Answer from the drawing. Dimensions are ordinates in mm from the lowest x, y and z of the part. Round coordinates to 2 decimals unless told otherwise and drop trailing zeros. Loops run counter-clockwise (first coordinate to the right, second up) from the corner with the lowest first, then second, coordinate; pieces in that order, holes last.
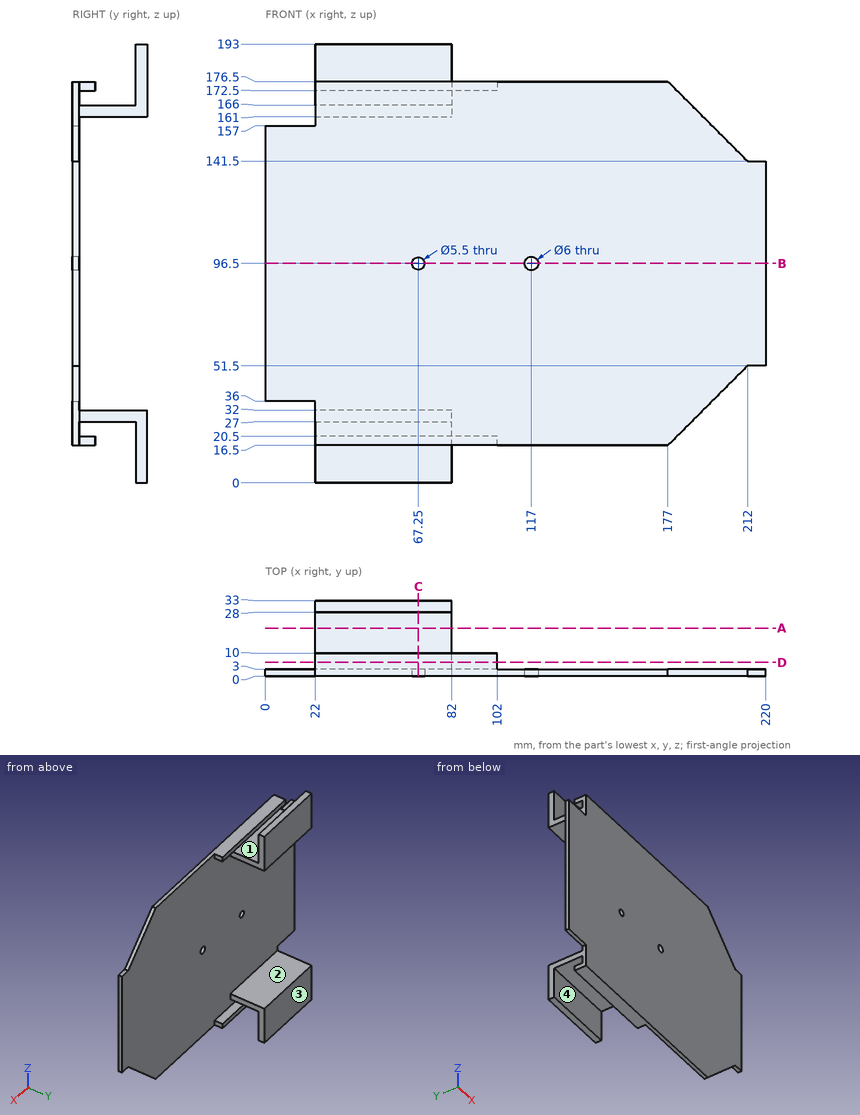
Item 1: Straight lines are drawn through the part: line 1 (Z direction, x = 40, y = 6); line 2 (X direction, y = 2, z = 96); line 3 (Z direction, x = 67.25, y = 1.4). For each, find the intervals that lie inside material, in ascending order.
Item 2: Each of these flat-tipped pins is pushed along its axis until it touches: P1, Ø1.5, axis at x = 217.5, y = 1, coming from the -Z side; P2, Ø1.5, axis at x = 215, y = 1, coming from the +Z side; P3, Ø5, axis at x = 130, y = 4, coming from the +Z side; P4, Ø5, axis at x = 117, z = 96.5, coming from the +Y side. Where does it stop, or does it pass through?
Item 3: Section C-C, the plane x = 67.25 is taken. Give the vertices of the cut face in (y, z), plus the area to 3 significant figures.
Item 4: Section D-D, the plane y = 6 is taken. Give the vertices of the cut face in (x, z), plus the area to 3 significant figures.
Item 5: Determine the mould class of the marked faces 1, 2, 3 and 4 for opening direction Y: pulls with the +Y half, pulls with the -Y half, needs draft (parallel to the pull), parting line crosses it, or undercut.
Item 6: Section B-B, the plane z = 96.5 is taken. Give the vertices of the cut face in (x, y).
Item 7: Section A-A, the plane y = 21 is taken. Give the vertices of the cut face in (x, z).
Answer below:
1. line 1: z = 16.5 to 20.5, 27 to 32, 161 to 166, 172.5 to 176.5
1. line 2: x = 0 to 64.55, 69.95 to 114.04, 119.96 to 220
1. line 3: z = 16.5 to 93.75, 99.25 to 176.5
2. P1: stops at z = 51.5
2. P2: stops at z = 141.5
2. P3: stops at z = 176.5
2. P4: passes through
3. outline: (0, 16.5) - (10, 16.5) - (10, 20.5) - (3, 20.5) - (3, 27) - (28, 27) - (28, 0) - (33, 0) - (33, 32) - (3, 32) - (3, 93.75) - (0, 93.75) - close; (0, 99.25) - (3, 99.25) - (3, 161) - (33, 161) - (33, 193) - (28, 193) - (28, 166) - (3, 166) - (3, 172.5) - (10, 172.5) - (10, 176.5) - (0, 176.5) - close
3. area: 1,090 mm2
4. outline: (22, 16.5) - (102, 16.5) - (102, 20.5) - (22, 20.5) - close; (22, 27) - (82, 27) - (82, 32) - (22, 32) - close; (22, 161) - (82, 161) - (82, 166) - (22, 166) - close; (22, 172.5) - (102, 172.5) - (102, 176.5) - (22, 176.5) - close
4. area: 1,240 mm2
5. face 1: undercut
5. face 2: needs draft
5. face 3: pulls with the +Y half
5. face 4: undercut
6. outline: (0, 0) - (64.5, 0) - (64.5, 3) - (0, 3) - close; (70, 0) - (114, 0) - (114, 3) - (70, 3) - close; (120, 0) - (220, 0) - (220, 3) - (120, 3) - close
7. outline: (22, 27) - (82, 27) - (82, 32) - (22, 32) - close; (22, 161) - (82, 161) - (82, 166) - (22, 166) - close
